```python
from build123d import *

# Parameters (mm, degrees)
SKETCH_R             = 1.5
PAD_DEPTH            = 3
CHAMFER_SIZE         = 1.5
SKETCH019_R          = 3
POCKET007_DEPTH      = 5
POCKET007_DEPTH_BACK = 100
SKETCH020_R          = 3
PAD006_DEPTH         = 4
PAD014_DEPTH         = 2
SKETCH021_R          = 1.45
POCKET008_DEPTH      = 10
POCKET008_DEPTH_BACK = 10
PAD018_DEPTH         = 6
PAD009_DEPTH         = 6.6788950282
FILLET_R             = 1
FILLET001_R          = 2
CHAMFER001_SIZE      = 0.2
SKETCH084_R          = 1.5
POCKET014_DEPTH      = 6.6798950282
CHAMFER004_SIZE      = 1.5
SKETCH092_R          = 1.45
POCKET018_DEPTH      = 28.6798950282
CHAMFER009_SIZE      = 0.4


with BuildPart() as part:
    # Sketch → Pad (new body)
    with BuildSketch(Plane.XY):
        with BuildLine():
            Line((-32, -44), (30.1435935394, -44))
            ThreePointArc((30.1435935394, -44), (31.4529008809, -43.511857892), (32.1230801767, -42.2857142857))
            ThreePointArc((42.2857142857, -32.1230801767), (35.5147186258, -35.5147186258), (32.1230801767, -42.2857142857))
            ThreePointArc((42.2857142857, -32.1230801767), (43.511857892, -31.4529008809), (44, -30.1435935394))
            Line((44, -30.1435935394), (44, 13))
            ThreePointArc((44, 13), (43.4142135624, 14.4142135624), (42, 15))
            Line((42, 15), (33.7448172036, 15))
            ThreePointArc((32.7448172036, 16), (33.0377104224, 15.2928932188), (33.7448172036, 15))
            Line((32.7448172036, 17), (32.7448172036, 16))
            ThreePointArc((32.7448172036, 17), (32.4519239848, 17.7071067812), (31.7448172036, 18))
            Line((24.7448172036, 18), (31.7448172036, 18))
            ThreePointArc((22.7448172036, 20), (23.3306036412, 18.5857864376), (24.7448172036, 18))
            Line((22.7448172036, 35), (22.7448172036, 20))
            ThreePointArc((22.7448172036, 35), (22.159030766, 36.4142135624), (20.7448172036, 37))
            Line((20.7448172036, 37), (-27, 37))
            ThreePointArc((-27, 37), (-30.5355339059, 35.5355339059), (-32, 32))
            Line((-32, 32), (-32, -44))
        make_face()
        with Locations((-14, 28)):
            Circle(SKETCH_R, mode=Mode.SUBTRACT)
        with Locations((0, 28)):
            Circle(SKETCH_R, mode=Mode.SUBTRACT)
        with Locations((0, -28)):
            Circle(SKETCH_R, mode=Mode.SUBTRACT)
        with Locations((-14, -28)):
            Circle(SKETCH_R, mode=Mode.SUBTRACT)
        with Locations((28, 14)):
            Circle(SKETCH_R, mode=Mode.SUBTRACT)
        with Locations((-28, -14)):
            Circle(SKETCH_R, mode=Mode.SUBTRACT)
        with Locations((-28, 0)):
            Circle(SKETCH_R, mode=Mode.SUBTRACT)
        with Locations((-28, 14)):
            Circle(SKETCH_R, mode=Mode.SUBTRACT)
        Polygon((9.8578643763, -18), (18, -9.8578643763), (18, 9.8578643763), (9.8578643763, 18), (-9.8578643763, 18), (-18, 9.8578643763), (-18, -9.8578643763), (-9.8578643763, -18), align=None, mode=Mode.SUBTRACT)
    extrude(amount=PAD_DEPTH)

    # Chamfer
    chamfer_edges = [part.edges().sort_by_distance(p)[0] for p in [
        (-1.5, -28, 3),
        (26.5, 14, 3),
        (-1.5, 28, 3),
        (-29.5, 0, 3),
    ]]
    chamfer(chamfer_edges, length=CHAMFER_SIZE)

    # Sketch019 (on Face1 of CopyPart__Feature008) → Pocket007 (cut, two sides)
    with BuildSketch(Plane(origin=(7.7448172036, 0, 2.4788950282), x_dir=(-1, 0, 0), z_dir=(0, 0, -1))) as pocket007_sk:
        with Locations((-4.0828427125, -30.8)):
            Circle(SKETCH019_R)
        Polygon((-23.7455844123, 2.8), (-17.3130471727, 2.8), (-10.2551827964, 9.8578643763), (4.5455844122, 9.8578643763), (4.5455844122, -18), (-3.2544155877, -25.8), (-23.7455844123, -25.8), (-27.8, -21.7455844123), (-27.8, -1.2544155877), align=None)
    extrude(amount=-POCKET007_DEPTH, mode=Mode.SUBTRACT)
    extrude(pocket007_sk.sketch, amount=POCKET007_DEPTH_BACK, mode=Mode.SUBTRACT)

    # Sketch020 (on Face1 of CopyPart__Feature008001) → Pad006 (join)
    with BuildSketch(Plane(origin=(7.7448172036, 0, 4.9788950282), x_dir=(-1, 0, 0), z_dir=(0, 0, -1))):
        with Locations((-11, 31)):
            Circle(SKETCH020_R)
        with Locations((-30, -24)):
            Circle(SKETCH020_R)
        with Locations((30, -24)):
            Circle(SKETCH020_R)
    extrude(amount=PAD006_DEPTH)

    # Sketch037 (on Face4 of Pad006) → Pad014 (join)
    with BuildSketch(Plane.XY.offset(3)):
        with BuildLine():
            ThreePointArc((-22.2551827964, -28), (-18.2551827964, -24), (-22.2551827964, -20))
            Line((-22.2551827964, -20), (-32, -20))
            Line((-32, -20), (-32, -28))
            Line((-32, -28), (-22.2551827964, -28))
        make_face()
        with BuildLine():
            ThreePointArc((-22, 22), (-19.1715728753, 23.1715728753), (-18, 26))
            Line((-18, 28), (-18, 26))
            ThreePointArc((-14, 32), (-16.8284271247, 30.8284271247), (-18, 28))
            Line((-14, 32), (0, 32))
            ThreePointArc((4, 28), (2.8284271247, 30.8284271247), (0, 32))
            Line((4, 28), (4, 27))
            ThreePointArc((4, 27), (4.5857864376, 25.5857864376), (6, 25))
            Line((20.7448172036, 25), (6, 25))
            ThreePointArc((20.7448172036, 25), (22.159030766, 25.5857864376), (22.7448172036, 27))
            Line((22.7448172036, 35), (22.7448172036, 27))
            ThreePointArc((22.7448172036, 35), (22.159030766, 36.4142135624), (20.7448172036, 37))
            Line((20.7448172036, 37), (-27, 37))
            ThreePointArc((-27, 37), (-30.5355339059, 35.5355339059), (-32, 32))
            Line((-32, 32), (-32, 22))
            Line((-32, 22), (-22, 22))
        make_face()
        with BuildLine():
            ThreePointArc((37.7448172036, -21), (35.6234968601, -21.8786796564), (34.7448172036, -24))
            Line((34.7448172036, -32.0265993723), (34.7448172036, -24))
            ThreePointArc((34.7448172036, -32.0265993723), (35.7632137629, -33.7691419644), (37.7812718888, -33.7370851763))
            ThreePointArc((42.2857142857, -32.1230801767), (39.9522314637, -32.7032938484), (37.7812718888, -33.7370851763))
            ThreePointArc((42.2857142857, -32.1230801767), (43.511857892, -31.4529008809), (44, -30.1435935394))
            Line((44, -23), (44, -30.1435935394))
            ThreePointArc((44, -23), (43.4142135624, -21.5857864376), (42, -21))
            Line((37.7448172036, -21), (42, -21))
        make_face()
    extrude(amount=PAD014_DEPTH)

    # Sketch021 → Pocket008 (cut, two sides)
    with BuildSketch(Plane.XY) as pocket008_sk:
        with Locations((18.7448172036, 31)):
            Circle(SKETCH021_R)
        with Locations((37.7448172036, -24)):
            Circle(SKETCH021_R)
        with Locations((-22.2551827964, -24)):
            Circle(SKETCH021_R)
    extrude(amount=-POCKET008_DEPTH, mode=Mode.SUBTRACT)
    extrude(pocket008_sk.sketch, amount=POCKET008_DEPTH_BACK, mode=Mode.SUBTRACT)

    # Sketch047 (on Face1 of ShapeBinder003) → Pad018 (join)
    with BuildSketch(Plane(origin=(0, -38.0039418631, 0), x_dir=(-1, 0, 0), z_dir=(0, 1, 0))):
        with BuildLine():
            Line((5.016001945, 11.5), (10.0080009725, 11.5))
            ThreePointArc((10.0080009725, 11.5), (18.5080009725, 3.0000209515), (27.0080009725, 11.5))
            Line((27.0080009725, 11.5), (32, 11.5))
            Line((32, 11.5), (32, 0))
            Line((32, 0), (5.016001945, 0))
            Line((5.016001945, 0), (5.016001945, 11.5))
        make_face()
    extrude(amount=-PAD018_DEPTH)

    # Sketch025 → Pad009 (join)
    with BuildSketch(Plane.XY):
        with BuildLine():
            Line((-2.8599687425, 41.8047859461), (-20.8599687425, 41.8047859461))
            ThreePointArc((-20.8599687425, 41.8047859461), (-32.8807840227, 36.8256012263), (-37.8599687425, 24.8047859461))
            Line((-37.8599687425, -21.9210564422), (-37.8599687425, 24.8047859461))
            ThreePointArc((-37.8599687425, -21.9210564422), (-36.3493363525, -30.4796550005), (-32, -38.0039418631))
            Line((-5.016001945, -38.0039418631), (-32, -38.0039418631))
            Line((-5.016001945, -38.0039418631), (-5.016001945, -36))
            Line((-5.016001945, -36), (-23.2551827964, -36))
            ThreePointArc((-28.2551827964, -31), (-26.7907167023, -34.5355339059), (-23.2551827964, -36))
            Line((-28.2551827964, -31), (-28.2551827964, -17.4906849959))
            ThreePointArc((-28.2551827964, -10.5093150041), (-31.5, -14), (-28.2551827964, -17.4906849959))
            Line((-28.2551827964, -10.5093150041), (-28.2551827964, -3.4906849959))
            ThreePointArc((-28.2551827964, 3.4906849959), (-31.5, 0), (-28.2551827964, -3.4906849959))
            Line((-28.2551827964, 3.4906849959), (-28.2551827964, 10.5093150041))
            ThreePointArc((-28.2551827964, 17.4906849959), (-31.5, 14), (-28.2551827964, 10.5093150041))
            Line((-28.2551827964, 17.4906849959), (-28.2551827964, 31))
            ThreePointArc((-23.2551827964, 36), (-26.7907167023, 34.5355339059), (-28.2551827964, 31))
            Line((9.4711954522, 36), (-23.2551827964, 36))
            ThreePointArc((9.4711954522, 36), (3.9545956287, 40.2810324358), (-2.8599687425, 41.8047859461))
        make_face()
    extrude(amount=PAD009_DEPTH)

    # Fillet
    fillet_edges = [part.edges().sort_by_distance(p)[0] for p in [
        (-28.255183, -20, 4),
        (-28.255183, -28, 4),
    ]]
    fillet(fillet_edges, radius=FILLET_R)

    # Fillet001
    fillet001_edges = [part.edges().sort_by_distance(p)[0] for p in [
        (9.857864, 18, 1.5),
        (35.544817, -21.745584, 1.5),
        (25.057864, 2.8, 1.5),
        (31.490402, -25.8, 1.5),
        (3.199233, -18, 1.5),
    ]]
    fillet(fillet001_edges, radius=FILLET001_R)

    # Chamfer001
    chamfer001_edges = [part.edges().sort_by_distance(p)[0] for p in [
        (7.392126, -22.192893, 3),
    ]]
    chamfer(chamfer001_edges, length=CHAMFER001_SIZE)

    # Sketch084 (on Face77 of Chamfer001) → Pocket014 (cut, through all)
    with BuildSketch(Plane.XY.offset(6.6788950282)):
        with Locations((-31.2551827964, 28)):
            Circle(SKETCH084_R)
    extrude(amount=-POCKET014_DEPTH, mode=Mode.SUBTRACT)

    # Chamfer004
    chamfer004_edges = [part.edges().sort_by_distance(p)[0] for p in [
        (-15.5, 28, 3),
        (-15.5, -28, 3),
        (-29.5, 14, 3),
        (-29.5, -14, 3),
    ]]
    chamfer(chamfer004_edges, length=CHAMFER004_SIZE)

    # Sketch092 (on Face1 of CopyCopyPad022) → Pocket018 (cut, through all)
    with BuildSketch(Plane.XY.offset(28.6788950282)):
        with Locations((-29, -41.0039418631)):
            Circle(SKETCH092_R)
        with Locations((-10.0080009725, -41.5039418631)):
            Circle(SKETCH092_R)
    extrude(amount=-POCKET018_DEPTH, mode=Mode.SUBTRACT)

    # Chamfer009
    chamfer009_edges = [part.edges().sort_by_distance(p)[0] for p in [
        (-32.755183, 28, 6.678895),
        (17.294817, 31, 5),
        (36.294817, -24, 5),
        (-23.705183, -24, 5),
        (-30.45, -41.003942, 11.5),
        (-8.982696, -42.529247, 11.5),
    ]]
    chamfer(chamfer009_edges, length=CHAMFER009_SIZE)


solid = part.part
```
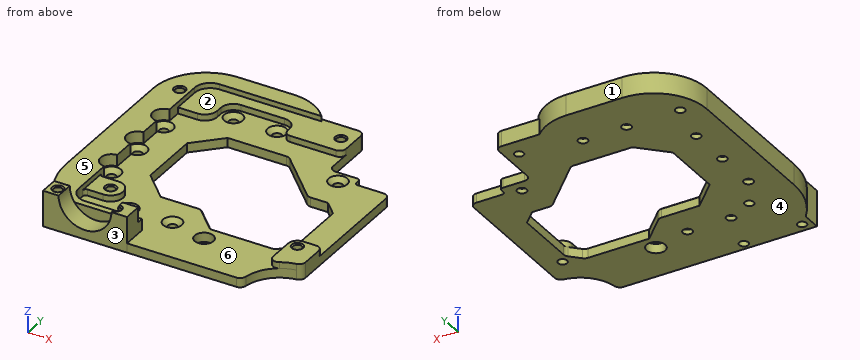
Can you work these out from the model? Positions are in its coordinate system, mm. Face numbers are marked on the shaded views. A direction names the side the tool comes from. Round coordinates to 2 decimals unless told otherwise and drop trailing zeros. Order: outer loops, then holes, each group sorted by start corner. A loop starts at its lowest first (then second) coordinate and runs counter-clockwise, first axis right, second up. Notation, with made-up numbers: (5.5, 85.5) -> (25.5, 85.5) arc R24 cw to (25.5, 97.5) -> close; hole circle Ø9 at (40, 28). An arc over 180 degrees is marked (long way). Return JSON: item names as keys, results as strings. Group by question number.
1. If we section it at B-B, the plane x = 28: Write out the boundary of the cut face in (y, z).
2. If we section it at A-A, the plane z = 9: Write out the boundary of the cut face in (x, y), then the cut area to 3 significant figures.
3. Will these pins go through, and if not, where does the flat tip stop? pin 1 (2.5 mm diameter, centred on x = 37.5, z = 1, fed in from +Y); pin 2 (2.5 mm diameter, centred on x = -28, y = 0, fed in from -Z); pin 3 (2 mm diameter, centred on x = -27.5, z = 4, fed in from +Y); pin 4 (4 mm diameter, centred on x = 0, y = 28, fed in from +Z).
4. If we section it at D-D, the plane x = 13.5: Write out the boundary of the cut face in (y, z), then the cut area to 3 significant figures.
5. I need wall thicknesses on line 1 (Y direction, x = 28, z = 0.95); line 2 (X direction, y = -24, z = 1.3); line 3 (X direction, y = -21, z = 5.5). Which ranges of each line are inside material? Lowest first, please. Write a range as [from, to].
6. We'd pull the mould along Y, two halves only. Please class the marked faces 1, 2 and 3: released by +Y, released by -Y, zero draft, split by the parting line, or undercut.
7. Which directions (+Z, -Z, +X, -X, +Y, -Y) give clear straight access to the entire face, cutting with the end or side of a thin tool? Please do the marked faces 4, 5 and 6.
8. If we section it at C-C, the plane y = 0: Write out the boundary of the cut face in (x, z).
Output values:
{
 "1": {"outline": "(-44, 0) -> (-25.8, 0) -> (-25.8, 3) -> (-44, 3) -> close; (2.8, 0) -> (12.5, 0) -> (12.5, 1.5) -> (11, 3) -> (2.8, 3) -> close; (15.5, 0) -> (18, 0) -> (18, 3) -> (17, 3) -> (15.5, 1.5) -> close"},
 "2": {"outline": "(-32, -44) -> (-26.63, -44) -> (-26.63, -38) -> (-32, -38) -> close; (-10.38, -44) -> (-5.02, -44) -> (-5.02, -38) -> (-10.38, -38) -> (-10.38, -40.1) arc R1.45 cw (long way) to (-10.38, -42.9) -> close; hole circle Ø2.9 at (-29, -41)", "area": "53.4 mm²"},
 "3": {"pin 1": "y = 15", "pin 2": "through", "pin 3": "y = 40.84", "pin 4": "z = 2"},
 "4": {"outline": "(-44, 0) -> (-33.29, 0) -> (-33.29, 3) -> (-44, 3) -> close; (-28.31, 0) -> (-25.8, 0) -> (-25.8, 3) -> (-28.31, 3) -> close; (14.36, 0) -> (37, 0) -> (37, 5) -> (25, 5) -> (25, 3) -> (14.36, 3) -> close", "area": "132 mm²"},
 "5": {"line 1": "[-44, -25.8], [2.8, 12.5], [15.5, 18]", "line 2": "[-37.77, -23.71], [-20.81, 9.2], [33.29, 36.29], [39.19, 44]", "line 3": "[-37.86, -28.26]"},
 "6": {"face 1": "released by +Y", "face 2": "undercut", "face 3": "released by -Y"},
 "7": {"face 4": "-Z, +X, -X, +Y, -Y", "face 5": "+Z, +X, -X, +Y", "face 6": "+Z"},
 "8": {"outline": "(-37.86, 0) -> (-29.5, 0) -> (-29.5, 1.5) -> (-31, 3) -> (-31.5, 3) -> (-31.5, 6.68) -> (-37.86, 6.68) -> close; (-26.5, 0) -> (-18, 0) -> (-18, 3) -> (-25, 3) -> (-26.5, 1.5) -> close; (34.29, 0) -> (44, 0) -> (44, 3) -> (34.29, 3) -> close"}
}
